```python
from build123d import *

# Parameters (mm, degrees)
SKETCH2_W                    = 25.4
SKETCH2_H                    = 50.8
BOSS_EXTRUDE1_DEPTH          = 50.8
SKETCH3_W                    = 50.8
SKETCH3_H                    = 44.45
CUT_EXTRUDE1_DEPTH           = 63.217039467
SKETCH4_R                    = 6.35
CUT_EXTRUDE2_DEPTH           = 73.955945611
F_10_0_1935_DIAMETER_HOLE2_D = 4.9149
SKETCH9_W                    = 19.05
SKETCH9_H                    = 44.45
CUT_EXTRUDE3_DEPTH           = 106.494123059


with BuildPart() as part:
    # Sketch2 → Boss-Extrude1 (new, symmetric)
    with BuildSketch(Plane.XY):
        Rectangle(SKETCH2_W, SKETCH2_H)
    extrude(amount=BOSS_EXTRUDE1_DEPTH, both=True)

    # Sketch3 → Cut-Extrude1 (cut, through all)
    with BuildSketch(Plane(origin=(12.7, 0, 0), x_dir=(0, 0, -1), z_dir=(1, 0, 0))):
        with Locations((-25.4, 0)):
            Rectangle(SKETCH3_W, SKETCH3_H)
    extrude(amount=-CUT_EXTRUDE1_DEPTH, mode=Mode.SUBTRACT)

    # Sketch4 → Cut-Extrude2 (cut, through all)
    with BuildSketch(Plane(origin=(0, 25.4, 0), x_dir=(1, 0, 0), z_dir=(0, 1, 0))):
        with Locations(Location((0, -38.1, 0), (0, 0, 270))):
            Circle(SKETCH4_R)
    extrude(amount=-CUT_EXTRUDE2_DEPTH, mode=Mode.SUBTRACT)

    # #10 (0.1935) Diameter Hole2 (through all)
    with Locations(Plane(origin=(12.7, 0, 0), x_dir=(0, 0, -1), z_dir=(1, 0, 0))):
        with Locations((12.7, 12.7), (38.1, 12.7), (12.7, -12.7), (38.1, -12.7)):
            Hole(F_10_0_1935_DIAMETER_HOLE2_D / 2)

    # Sketch9 → Cut-Extrude3 (cut, through all)
    with BuildSketch(Plane(origin=(0, 0, -50.8), x_dir=(-1, 0, 0), z_dir=(0, 0, -1))):
        Rectangle(SKETCH9_W, SKETCH9_H)
    extrude(amount=-CUT_EXTRUDE3_DEPTH, mode=Mode.SUBTRACT)


solid = part.part
```
The model under review builds one solid part; all positions refer to its coordinate system, in mm. A direction names the side the tool comes from. Give positions to 0.01 mm unless a question says otherwise; leave off trailing zeros. Write each loop counter-clockwise with the first axis right and the second up, starting at its lowest first coordinate (ties: lowest second). Pieces come first, ordered by that corner, then holes. Notation, with made-up numbers: (44, 27) -> (97, 27) arc R29 ccw to (97, 51) -> close; hole circle Ø2 at (-7.75, 15.25). An arc over 180 degrees is marked (long way). Answer in a Markdown table with one row per item.
1) Add section B-B on x = -7.5. State the section outline as (y, z) points (3 decimals).
Worked answers:
| item | result |
|---|---|
| outline | (-25.4, -50.8) -> (-22.225, -50.8) -> (-22.225, 50.8) -> (-25.4, 50.8) -> close; (22.225, -50.8) -> (25.4, -50.8) -> (25.4, 50.8) -> (22.225, 50.8) -> close |
2) Add section D-D on x = 0. State the section outline as (y, z) points (3 decimals), plus the area to 3 significant figures.
Worked answers:
| item | result |
|---|---|
| outline | (-25.4, -50.8) -> (-22.225, -50.8) -> (-22.225, 31.75) -> (-25.4, 31.75) -> close; (-25.4, 44.45) -> (-22.225, 44.45) -> (-22.225, 50.8) -> (-25.4, 50.8) -> close; (22.225, -50.8) -> (25.4, -50.8) -> (25.4, 31.75) -> (22.225, 31.75) -> close; (22.225, 44.45) -> (25.4, 44.45) -> (25.4, 50.8) -> (22.225, 50.8) -> close |
| area | 565 mm² |
3) Add section C-C on y = -12.7. State the section outline as (x, z) points (3 decimals), plus the area to 3 significant figures.
Worked answers:
| item | result |
|---|---|
| outline | (-12.7, -50.8) -> (-9.525, -50.8) -> (-9.525, -40.557) -> (-12.7, -40.557) -> close; (-12.7, -35.643) -> (-9.525, -35.643) -> (-9.525, -15.157) -> (-12.7, -15.157) -> close; (-12.7, -10.243) -> (-9.525, -10.243) -> (-9.525, 0) -> (-12.7, 0) -> close; (9.525, -50.8) -> (12.7, -50.8) -> (12.7, -40.557) -> (9.525, -40.557) -> close; (9.525, -35.643) -> (12.7, -35.643) -> (12.7, -15.157) -> (9.525, -15.157) -> close; (9.525, -10.243) -> (12.7, -10.243) -> (12.7, 0) -> (9.525, 0) -> close |
| area | 260 mm² |
4) Mouldability with a two-part tool opening along X and no side actions: class faces 1 (the flat face through (0, 22.225, 1)), 2 (the cylindrical face through (-11.13, -15.1, -13.23)), 3 (the flat face through (12.7, 0, -22)), 4 (the flat face through (-9.525, 0, -26)) as +X half, -X half, draft (parallel to the pull), parting line (faces both ways), or undercut.
Worked answers:
| item | result |
|---|---|
| face 1 | undercut |
| face 2 | draft |
| face 3 | +X half |
| face 4 | undercut |
5) Clearance check with flat-ended pins moving along their axes: P1, Ø4, axis at y = -12.7, z = -38.1, coming from the +X side; P2, Ø2.5, axis at x = 11.5, y = -9, coming from the +Z side. State where each tip first meets the part, or that it passes through.
Worked answers:
| item | result |
|---|---|
| P1 | through |
| P2 | z = 0 |
6) Add section A-A on z = -38.1. State the section outline as (x, y) points (3 decimals).
Worked answers:
| item | result |
|---|---|
| outline | (-12.7, -25.4) -> (12.7, -25.4) -> (12.7, -15.157) -> (9.525, -15.157) -> (9.525, -22.225) -> (-9.525, -22.225) -> (-9.525, -15.157) -> (-12.7, -15.157) -> close; (-12.7, -10.243) -> (-9.525, -10.243) -> (-9.525, 10.243) -> (-12.7, 10.243) -> close; (-12.7, 15.157) -> (-9.525, 15.157) -> (-9.525, 22.225) -> (9.525, 22.225) -> (9.525, 15.157) -> (12.7, 15.157) -> (12.7, 25.4) -> (-12.7, 25.4) -> close; (9.525, -10.243) -> (12.7, -10.243) -> (12.7, 10.243) -> (9.525, 10.243) -> close |
7) Tool access review of faces 5 (the flat face through (9.525, 0, -26)), 6 (the flat face through (-11, 0, 0)), 7 (the flat face through (0, -22.225, 1)): name each direction out of +Z, -Z, +X, -X, +Y, -Y from which nothing blocks a thin tool from reaching the whole face with its end or side.
Worked answers:
| item | result |
|---|---|
| face 5 | +Z, -Z |
| face 6 | +Z, +X, -X |
| face 7 | +Z |
8) For L1, parallel to Y at x = 11.2, z = -38.1; L2, parallel to Y at x = -5, z = -35.5 (3 decimals); L3, parallel to X at y = 10, z = -10 (3 decimals), list the stretches that pass through material, from the lowest coordinate up. Write a range as [from, to].
Worked answers:
| item | result |
|---|---|
| L1 | [-25.4, -15.16], [-10.24, 10.24], [15.16, 25.4] |
| L2 | [-25.4, -22.225], [22.225, 25.4] |
| L3 | [-12.7, -9.525], [9.525, 12.7] |
